Geometry: final body of the model. Coordinates: model frame, mm. Face numbers are marked on the shaded views. A direction names the side the tool comes from. Give positions to 0.01 mm unless a question says otherwise; leave off trailing zeros. Loops run counter-clockwise (first coordinate to the right, second up) from the corner with the lowest first, then second, coordinate; pieces in that order, holes last. Notation, with made-up numbers: (78.25, 80) - (108.25, 80) arc R27 ccw to (108.25, 104) - close; hole circle Ø5 at (37.25, -38.5). An arc over 180 degrees is marked (long way). Use one line per item in the form item = value.
```python
from build123d import *

# Parameters (mm, degrees)
CROQUIS1_W              = 140
CROQUIS1_H              = 64
SALIENTE_EXTRUIR1_DEPTH = 19
CROQUIS2_R              = 19
CROQUIS2_R_2            = 9.5
SALIENTE_EXTRUIR2_DEPTH = 19
SALIENTE_EXTRUIR3_DEPTH = 16
CROQUIS5_R              = 19
CROQUIS5_R_2            = 9.5
SALIENTE_EXTRUIR4_DEPTH = 19
SALIENTE_EXTRUIR5_START = -16
SALIENTE_EXTRUIR5_DEPTH = 16
SALIENTE_EXTRUIR6_DEPTH = 64
SALIENTE_EXTRUIR9_DEPTH = 18
CROQUIS14_R             = 16
CORTAR_EXTRUIR1_DEPTH   = 9
CROQUIS16_R             = 9.5
CORTAR_EXTRUIR2_DEPTH   = 19
CORTAR_EXTRUIR3_DEPTH   = 6
CORTAR_EXTRUIR4_DEPTH   = 187.944448389
CROQUIS19_R             = 6.5
CORTAR_EXTRUIR5_DEPTH   = 200.23943884
REDONDEO1_R             = 5


with BuildPart() as part:
    # Croquis1 → Saliente-Extruir1 (new body)
    with BuildSketch(Plane(origin=(0, 0, 0), x_dir=(1, 0, 0), z_dir=(0, 1, 0))):
        Rectangle(CROQUIS1_W, CROQUIS1_H)
    extrude(amount=SALIENTE_EXTRUIR1_DEPTH)



with BuildPart() as body_2:
    # Croquis2 → Saliente-Extruir2 (new body)
    with BuildSketch(Plane(origin=(37, 0, 0), x_dir=(0, 0, -1), z_dir=(1, 0, 0))):
        with Locations((0, 44)):
            Circle(CROQUIS2_R)
        with Locations((0, 44)):
            Circle(CROQUIS2_R_2, mode=Mode.SUBTRACT)
    extrude(amount=SALIENTE_EXTRUIR2_DEPTH)


with BuildPart() as part_1:
    add(part.part)

    add(body_2.part)  # Saliente-Extruir3 merges body 2
    # Croquis4 → Saliente-Extruir3 (add)
    with BuildSketch(Plane(origin=(37, 0, 0), x_dir=(0, 0, -1), z_dir=(1, 0, 0))):
        with BuildLine():
            ThreePointArc((19, 44), (0, 25), (-19, 44))
            Line((-19, 44), (-19, 19))
            Line((-19, 19), (19, 19))
            Line((19, 19), (19, 44))
        make_face()
    extrude(amount=SALIENTE_EXTRUIR3_DEPTH)



with BuildPart() as body_2_2:
    # Croquis5 → Saliente-Extruir4 (new body)
    with BuildSketch(Plane(origin=(8, 0, 0), x_dir=(0, 0, -1), z_dir=(1, 0, 0))):
        with Locations((0, 44)):
            Circle(CROQUIS5_R)
        with Locations((0, 44)):
            Circle(CROQUIS5_R_2, mode=Mode.SUBTRACT)
    extrude(amount=-SALIENTE_EXTRUIR4_DEPTH)


with BuildPart() as part_2:
    add(part_1.part)

    add(body_2_2.part)  # Saliente-Extruir5 merges body 2 2
    # Croquis6 → Saliente-Extruir5 (add)
    with BuildSketch(Plane(origin=(8, 0, 0), x_dir=(0, 0, -1), z_dir=(1, 0, 0)).offset(SALIENTE_EXTRUIR5_START)):
        with BuildLine():
            Line((19, 19), (19, 44))
            ThreePointArc((19, 44), (0, 25), (-19, 44))
            Line((-19, 44), (-19, 19))
            Line((-19, 19), (19, 19))
        make_face()
    extrude(amount=SALIENTE_EXTRUIR5_DEPTH)

    # Croquis7 → Saliente-Extruir6 (add)
    with BuildSketch(Plane.XY.offset(32)):
        Polygon((-70, 0), (-121.961524227, 90), (-105.507041555, 99.5), (-59.030344885, 19), (-70, 19), align=None)
    extrude(amount=-SALIENTE_EXTRUIR6_DEPTH)

    # Croquis9 → Saliente-Extruir9 (add)
    with BuildSketch(Plane(origin=(-69.461524227, 120.310889132, 0), x_dir=(0.8660254037844397, 0.4999999999999982, 0), z_dir=(-0.4999999999999983, 0.8660254037844398, 0))):
        with BuildLine():
            Line((-60.621778265, 32), (-9.621778265, 32))
            ThreePointArc((-9.621778265, 32), (22.378221735, 0), (-9.621778265, -32))
            Line((-9.621778265, -32), (-60.621778265, -32))
            Line((-60.621778265, -32), (-60.621778265, 32))
        make_face()
    extrude(amount=-SALIENTE_EXTRUIR9_DEPTH)

    # Croquis14 → Cortar-Extruir1 (cut)
    with BuildSketch(Plane(origin=(-69.461524227, 120.310889132, 0), x_dir=(0.8660254037844397, 0.4999999999999982, 0), z_dir=(-0.4999999999999983, 0.8660254037844398, 0))):
        with Locations(Location((-9.621778265, 0, 0), (0, 0, 180))):
            Circle(CROQUIS14_R)
    extrude(amount=-CORTAR_EXTRUIR1_DEPTH, mode=Mode.SUBTRACT)

    # Croquis16 → Cortar-Extruir2 (cut)
    with BuildSketch(Plane(origin=(-69.461524227, 120.310889132, 0), x_dir=(0.8660254037844397, 0.4999999999999982, 0), z_dir=(-0.4999999999999983, 0.8660254037844398, 0))):
        with Locations(Location((-9.621778265, 0, 0), (0, 0, 180))):
            Circle(CROQUIS16_R)
    extrude(amount=-CORTAR_EXTRUIR2_DEPTH, mode=Mode.SUBTRACT)

    # Croquis17 → Cortar-Extruir3 (cut)
    with BuildSketch(Plane(origin=(-69.461524227, 120.310889132, 0), x_dir=(0.8660254037844397, 0.4999999999999982, 0), z_dir=(-0.4999999999999983, 0.8660254037844398, 0))):
        with BuildLine():
            Line((-60.621778265, -11), (20.428180138, -11))
            ThreePointArc((20.428180138, -11), (22.378221735, 0), (20.428180138, 11))
            Line((20.428180138, 11), (-60.621778265, 11))
            Line((-60.621778265, 11), (-60.621778265, -11))
        make_face()
    extrude(amount=-CORTAR_EXTRUIR3_DEPTH, mode=Mode.SUBTRACT)

    # Croquis18 → Cortar-Extruir4 (cut, through all)
    with BuildSketch(Plane(origin=(-69.461524227, 120.310889132, 0), x_dir=(0.8660254037844397, 0.4999999999999982, 0), z_dir=(-0.4999999999999983, 0.8660254037844398, 0))):
        Polygon((-60.621778265, 21), (-54.621778265, 17.535898385), (-54.621778265, -17.535898385), (-60.621778265, -21), align=None)
    extrude(amount=-CORTAR_EXTRUIR4_DEPTH, mode=Mode.SUBTRACT)

    # Croquis19 → Cortar-Extruir5 (cut, through all)
    with BuildSketch(Plane(origin=(-47.303847577, -27.310889132, 0), x_dir=(0, 0, 1), z_dir=(-0.8660254037844396, -0.4999999999999983, 0))):
        with Locations(Location((0, 104.923048454, 0), (0, 0, 270))):
            Circle(CROQUIS19_R)
        with Locations(Location((0, 75.923048454, 0), (0, 0, 270))):
            Circle(CROQUIS19_R)
    extrude(amount=-CORTAR_EXTRUIR5_DEPTH, mode=Mode.SUBTRACT)

    # Redondeo1
    redondeo1_edges = [part_2.edges().sort_by_distance(p)[0] for p in [
        (-59.030344885, 19, 0),
        (-96.507041555, 83.911542732, 0),
    ]]
    fillet(redondeo1_edges, radius=REDONDEO1_R)


solid = part_2.part
```
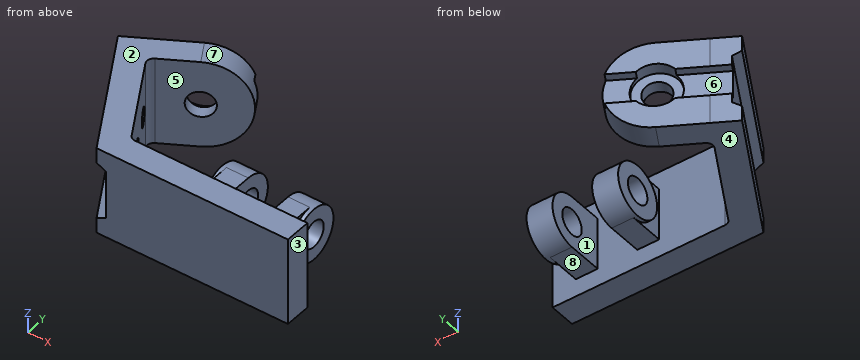
(1) Cut plane C-C (y = 17). Return the cut outline in (x, z).
Solution:
outline = (-79.81, -32) - (70, -32) - (70, 32) - (-79.81, 32) - (-79.81, 21) - (-72.89, 17.54) - (-72.89, -17.54) - (-79.81, -21) - close
(2) Cut plane A-A (x = 2). Return the cut outline in (y, z), plus the area to 3 significant figures.
Solution:
outline = (0, -32) - (19, -32) - (19, -19) - (44, -19) arc R19 ccw to (44, 19) - (19, 19) - (19, 32) - (0, 32) - close; hole circle Ø19 at (44, 0)
area = 2,450 mm2
(3) Cut plane D-D (z = 0). Give the number of separate pieces and of enclosed holes in the cut face, plus the area to 3 significant figures.
Solution:
separate_pieces = 6
enclosed_holes = 0
area = 4,800 mm2
(4) Access query for the marked faces 4, 5, 6, 7 and 8. Directions: +Z, -Z, +X, -X, +Y, -Y. A direction counts if a zero-diameter tool reaches every point of the face in a straight line with its end or side. Return the directions, or none.
Solution:
face_4 = -Z, +X, -X, +Y, -Y
face_5 = +Z, -Z, +X
face_6 = -X, +Y
face_7 = +X, +Y
face_8 = -Z, +X, +Y
(5) Pin query (flat end, axial travel): P1, Ø6, axis at x = -88, z = 25, coming from the -Y side; P2, Ø4.5, axis at x = -63, y = 119.5, coming from the -Z side; P3, Ø11.5, axis at y = 43, z = 8.5, coming from the -X side; P4, Ø10, axis at x = -60, z = 7.5, coming from the -Y side. Return the tip coordinate at first contact, or that it passes through.
Solution:
P1 = 25.98
P2 = -29.43
P3 = -91.22
P4 = 0
(6) Pull-direction query (X, two-part tool) for the marked faces 1, 2 and 3; classes: released by +X, released by -X, zero draft, split by the parting line, or undercut.
Solution:
face_1 = undercut
face_2 = zero draft
face_3 = released by +X
(7) Cut plane B-B (z = -25). Return the cut outline in (x, y), plus the area to 3 significant figures.
Solution:
outline = (-121.96, 90) - (-70, 0) - (70, 0) - (70, 19) - (-56.14, 19) arc R5 cw to (-60.47, 21.5) - (-94.01, 79.58) arc R5 cw to (-92.18, 86.41) - (-51.5, 109.9) - (-60.5, 125.49) - close
area = 5,370 mm2
(8) Material intervals for L1, parallel to Y at x = 49.5, z = 0; L2, parallel to Y at x = -33, z = -10; L3, parallel to Y at x = -53, z = -15, sorted ascending. Write a range as from..to.
Solution:
L1 = 0..34.5, 53.5..63
L2 = 0..19
L3 = 0..19, 109.03..129.09
